For this review, use the dimensioned drawing (mm, ordinates from the lowest corner) and the shaded views. A direction names the side the tool comes from. Give positions to 0.01 mm unless a question says otherwise; leave off trailing zeros. Order: outer loops, then holes, each group sorted by start corner. A loop starts at its lowest first (then second) coordinate and runs counter-clockwise, first axis right, second up. Notation, with made-up numbers: (89.25, 48) -> (122.25, 48) arc R12 ccw to (122.25, 65) -> close; hole circle Ø7 at (3.5, 84.5). An arc over 180 degrees is marked (long way). Return JSON: item names as keys, results as strings.
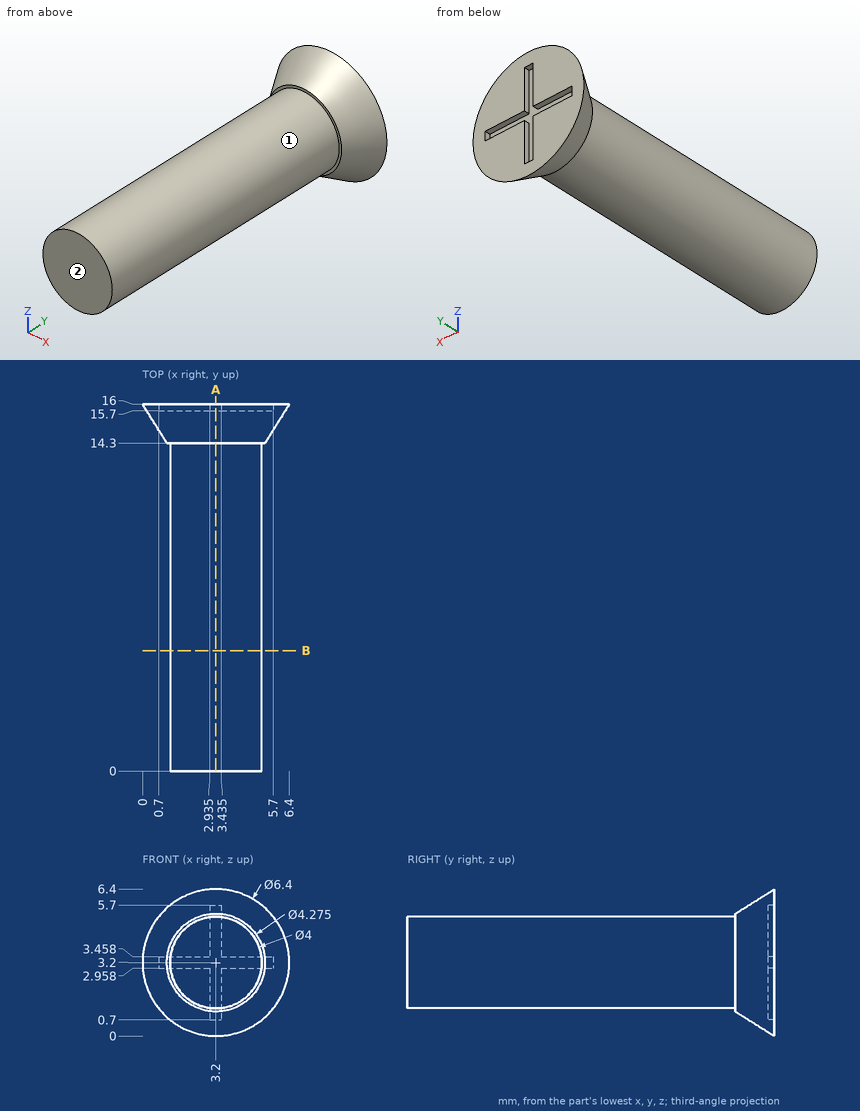
Item 1: Add section B-B (y = 5.25). Give the boundary of the cut face in (x, z).
Result set:
{"outline": "circle Ø4 at (3.2, 3.2)"}
Item 2: Wall thickness on L1, parallel to Y at x = 1.5, z = 3; L2, parallel to Z at x = 3.75, y = 11.25; L3, parallel to Y at x = 0.75, z = 2.5 (1 decimal): over which ranges is each line inside the solid? List them lowest first. Write a range as [from, to].
Result set:
{"L1": "y = [0, 15.7]", "L2": "z = [1.28, 5.12]", "L3": "y = [15, 16]"}
Item 3: For pin 1 (3 mm diameter, centred on x = 5, y = 10, fed in from -Z); pin 2 (2 mm diameter, centred on y = 14, z = 3.5, fed in from +X) (1 decimal), all flat-tipped, find the tip position at first contact; note any pin that passes through.
Result set:
{"pin 1": "stops at z = 1.22", "pin 2": "stops at x = 5.8"}
Item 4: Add section A-A (x = 3.2). Give the boundary of the cut face in (y, z).
Result set:
{"outline": "(0, 1.2) -> (14.3, 1.2) -> (14.3, 1.06) -> (16, 0) -> (16, 0.7) -> (15.7, 0.7) -> (15.7, 5.7) -> (16, 5.7) -> (16, 6.4) -> (14.3, 5.34) -> (14.3, 5.2) -> (0, 5.2) -> close"}
Item 5: Machinability: for the marked faces 1 and 2, which of the approach directions +Z, -Z, +X, -X, +Y, -Y give a long, thin tool a straight path to every point of the face, cutting with its end or side? Answer none if there is none.
Result set:
{"face 1": "-Y", "face 2": "+Z, -Z, +X, -X, -Y"}
